Verification items for the finished model (mm, model axes). A direction names the side the tool comes from. Coordinates: 2 decimals unless noted, no trailing zeros. Order: outer loops, then holes, each group sorted by start corner. A loop starts at its lowest first (then second) coordinate and runs counter-clockwise, first axis right, second up. Notation, with made-up numbers: M 71.5,87.5 L 106.5,87.5 A18 ccw 106.5,122.5 Z; hole C 7.25,2.5 d3. An arc over 180 degrees is marked long. Return JSON: item names as keys, results as strings.
```python
from build123d import *

# Parameters (mm, degrees)
EXTRUDE_2_DEPTH     = 10
SKETCH_4_R          = 1.45
CUT_EXTRUDE_1_DEPTH = 263.163594727
SKETCH_6_R          = 2.3
CUT_EXTRUDE_3_DEPTH = 4.5
SKETCH_11_R         = 1.45
CUT_EXTRUDE_4_DEPTH = 6.5
SKETCH_12_R         = 1.45
CUT_EXTRUDE_5_DEPTH = 10


with BuildPart() as part:
    # 草图2 → 凸台-拉伸2 (new body)
    with BuildSketch(Plane(origin=(0, 0, 0), x_dir=(1, 0, 0), z_dir=(0, 1, 0))):
        Polygon((0, 223), (0, 153), (-47.48, 153), (-47.48, 70), (0, 70), (0, 0), (90, 0), (90, 70), (137.48, 70), (137.48, 153), (90, 153), (90, 223), align=None)
    extrude(amount=EXTRUDE_2_DEPTH)

    # 草图4 → 切除-拉伸1 (cut, through all)
    with BuildSketch(Plane(origin=(0, 10, 0), x_dir=(1, 0, 0), z_dir=(0, 1, 0))):
        with Locations(Location((-41.98, 121.93, 0), (0, 0, 270))):
            Circle(SKETCH_4_R)
        with Locations(Location((-41.98, 102.68, 0), (0, 0, 270))):
            Circle(SKETCH_4_R)
        with Locations(Location((-31.06, 102.68, 0), (0, 0, 270))):
            Circle(SKETCH_4_R)
        with Locations(Location((-31.06, 121.93, 0), (0, 0, 270))):
            Circle(SKETCH_4_R)
    cut_extrude_1 = extrude(amount=-CUT_EXTRUDE_1_DEPTH, mode=Mode.SUBTRACT)

    # 镜向1: 切除-拉伸1 across plane
    add(cut_extrude_1.mirror(Plane(origin=(45, 0, 0), x_dir=(0, 0, 1), z_dir=(1, 0, 0))), mode=Mode.SUBTRACT)

    # 草图6 → 切除-拉伸3 (cut)
    with BuildSketch(Plane(origin=(0, 10, 0), x_dir=(1, 0, 0), z_dir=(0, 1, 0))):
        with Locations(Location((-41.98, 121.93, 0), (0, 0, 270))):
            Circle(SKETCH_6_R)
        with Locations(Location((-31.06, 121.93, 0), (0, 0, 270))):
            Circle(SKETCH_6_R)
        with Locations(Location((-41.98, 102.68, 0), (0, 0, 270))):
            Circle(SKETCH_6_R)
        with Locations(Location((-31.06, 102.68, 0), (0, 0, 270))):
            Circle(SKETCH_6_R)
    cut_extrude_3 = extrude(amount=-CUT_EXTRUDE_3_DEPTH, mode=Mode.SUBTRACT)

    # 镜向3: 切除-拉伸3 across plane
    add(cut_extrude_3.mirror(Plane(origin=(45, 0, 0), x_dir=(0, 0, 1), z_dir=(1, 0, 0))), mode=Mode.SUBTRACT)

    # 草图11 → 切除-拉伸4 (cut)
    with BuildSketch(Plane.XZ):
        with Locations(Location((33.98, -96.5, 0), (0, 0, 270))):
            Circle(SKETCH_11_R)
        with Locations(Location((13.98, -96.5, 0), (0, 0, 270))):
            Circle(SKETCH_11_R)
        with Locations(Location((33.98, -126.5, 0), (0, 0, 270))):
            Circle(SKETCH_11_R)
        with Locations(Location((13.98, -126.5, 0), (0, 0, 270))):
            Circle(SKETCH_11_R)
    cut_extrude_4 = extrude(amount=-CUT_EXTRUDE_4_DEPTH, mode=Mode.SUBTRACT)

    # 镜向4: 切除-拉伸4 across plane
    add(cut_extrude_4.mirror(Plane(origin=(45, 0, 0), x_dir=(0, 0, 1), z_dir=(1, 0, 0))), mode=Mode.SUBTRACT)

    # 草图12 → 切除-拉伸5 (cut)
    with BuildSketch(Plane(origin=(0, 10, 0), x_dir=(1, 0, 0), z_dir=(0, 1, 0))):
        with Locations(Location((61, 36, 0), (0, 0, 270))):
            Circle(SKETCH_12_R)
        with Locations(Location((29, 36, 0), (0, 0, 270))):
            Circle(SKETCH_12_R)
        with Locations(Location((29, 4, 0), (0, 0, 270))):
            Circle(SKETCH_12_R)
        with Locations(Location((61, 4, 0), (0, 0, 270))):
            Circle(SKETCH_12_R)
    extrude(amount=-CUT_EXTRUDE_5_DEPTH, mode=Mode.SUBTRACT)


solid = part.part
```
Q1. Tool access check on faces 1 (the face through (-23, 5, -153)), 2 (the face through (122.46, 7.781, -104.505)), 3 (the face through (90, 5, -35)), 4 (the face through (-24, 5, -70)). Record the directions out of +Z, -Z, +X, -X, +Y, -Y that give a thin tool (end or side, any length) a straight path to the whole face; none if there is none.
Values:
{"face 1": "-Z, -X, +Y, -Y", "face 2": "+Y", "face 3": "+Z, +X, +Y, -Y", "face 4": "+Z, -X, +Y, -Y"}
Q2. Cross-section at C-C, the plane z = -157.5. Record the boundary of the cut face in (x, y), and give its area (3 significant figures).
Values:
{"outline": "M 0,0 L 90,0 L 90,10 L 0,10 Z", "area": "900 mm^2"}
Q3. Go/stop test with flat-tipped pins: pin 1 (0.9 mm diameter, centred on x = 34, z = -97, fed in from -Y); pin 2 (5 mm diameter, centred on x = -17.5, y = 3.5, fed in from -Z). Record where each tip stops, or that it passes through.
Values:
{"pin 1": "y = 6.5", "pin 2": "z = -153"}
Q4. Material ranges on line 1 along X through (y, z) = (3, -36); line 2 along Z through (x, y) = (14, 2.5); line 3 along X through (y, z) = (4, -96.5), recorded low to high.
Values:
{"line 1": "0 to 27.55, 30.45 to 59.55, 62.45 to 90", "line 2": "-223 to -127.95, -125.05 to -97.95, -95.05 to 0", "line 3": "-47.48 to 12.53, 15.43 to 32.53, 35.43 to 54.57, 57.47 to 74.57, 77.47 to 137.48"}
Q5. Draft check along X on faces 5 (the face through (90, 5, -188)), 6 (the face through (114, 5, -153)), 7 (the face through (132, 5.5, -101)). Enter one of: pulls with the +X half, pulls with the -X half, needs draft (parallel to the pull), parting line crosses it, or undercut.
Values:
{"face 5": "pulls with the +X half", "face 6": "needs draft", "face 7": "undercut"}
Q6. Cross-section at A-A, the plane y = 8.25. State how many separate pieces and enclosed holes the cut face has, and give its area (3 significant figures).
Values:
{"separate pieces": "1", "enclosed holes": "12", "area": "27,800 mm^2"}
Q7. Cross-section at B-B, the plane x = -8. Record the boundary of the cut face in (y, z).
Values:
{"outline": "M 0,-153 L 10,-153 L 10,-70 L 0,-70 Z"}
